```python
from build123d import *

# Parameters (mm, degrees)
SKETCH1_W                = 2.5
SKETCH1_H                = 2.25
BOSS_EXTRUDE1_DEPTH      = 1.25
BOSS_EXTRUDE2_DEPTH      = 3.35
BOSS_EXTRUDE2_DEPTH_BACK = 6.35
SKETCH2_W                = 0.65
SKETCH2_H                = 0.65
SKETCH3_W                = 0.65
SKETCH3_H                = 0.65
BOSS_EXTRUDE3_DEPTH      = 0.5
BOSS_EXTRUDE3_TAPER      = 20
SKETCH7_W                = 0.65
SKETCH7_H                = 0.65
BOSS_EXTRUDE6_DEPTH      = 0.5
BOSS_EXTRUDE6_TAPER      = 20


with BuildPart() as part:
    # Sketch1 → Boss-Extrude1 (new, symmetric)
    with BuildSketch(Plane.XY):
        Rectangle(SKETCH1_W, SKETCH1_H)
    extrude(amount=BOSS_EXTRUDE1_DEPTH, both=True)

    # Sketch2 → Boss-Extrude2 (add, two sides: drawn at the far end of the back side and taken through both)
    with BuildSketch(Plane.XY.offset(-BOSS_EXTRUDE2_DEPTH_BACK)):
        Rectangle(SKETCH2_W, SKETCH2_H)
    extrude(amount=BOSS_EXTRUDE2_DEPTH + BOSS_EXTRUDE2_DEPTH_BACK)

    # Sketch3 → Boss-Extrude3 (add)
    with BuildSketch(Plane(origin=(0, 0, -6.35), x_dir=(-1, 0, 0), z_dir=(0, 0, -1))):
        Rectangle(SKETCH3_W, SKETCH3_H)
    extrude(amount=BOSS_EXTRUDE3_DEPTH, taper=BOSS_EXTRUDE3_TAPER)

    # Sketch7 → Boss-Extrude6 (add)
    with BuildSketch(Plane.XY.offset(3.35)):
        Rectangle(SKETCH7_W, SKETCH7_H)
    extrude(amount=BOSS_EXTRUDE6_DEPTH, taper=BOSS_EXTRUDE6_TAPER)


solid = part.part
```
CAD build for the part. Positions are in the model's coordinates, mm. Give positions to 0.01 mm unless a question says otherwise; leave off trailing zeros. Loops run counter-clockwise (first coordinate to the right, second up) from the corner with the lowest first, then second, coordinate; pieces in that order, holes last. Notation, with made-up numbers: (-33.5, 13) -> (-18.5, 13) arc R20 cw to (-18.5, 30) -> close; hole circle Ø1 at (67, -19.75). An arc over 180 degrees is marked (long way). Use a Markdown table: item, result.
1. Slice it at B-B (z = -4.25). List the corners of the cut face in (x, y) (3 decimals), plus the area to 4 significant figures.
Check result:
| item | result |
|---|---|
| outline | (-0.325, -0.325) -> (0.325, -0.325) -> (0.325, 0.325) -> (-0.325, 0.325) -> close |
| area | 0.4225 mm^2 |
2. Wall check: L1, parallel to Z at x = -0.15, y = 0.7; L2, parallel to Y at x = -0.1, z = 3 (3 decimals). Give the ranges that are in metal, low to high. Write a range as [from, to].
Check result:
| item | result |
|---|---|
| L1 | z = [-1.25, 1.25] |
| L2 | y = [-0.325, 0.325] |
3. Flat gauge pins, fed straight in: pin 1 (0.5 mm diameter, centred on y = 0, z = -4.5, fed in from -X) (3 decimals); pin 2 (0.7 mm diameter, centred on x = 0, z = 2.5, fed in from -Y) (3 decimals). Where does each tip first touch, or does it go through?
Check result:
| item | result |
|---|---|
| pin 1 | stops at x = -0.325 |
| pin 2 | stops at y = -0.325 |
4. Slice it at A-A (y = 0.65). List the corners of the cut face in (x, z).
Check result:
| item | result |
|---|---|
| outline | (-1.25, -1.25) -> (1.25, -1.25) -> (1.25, 1.25) -> (-1.25, 1.25) -> close |
